Part model, mm, in its own coordinate system. A direction names the side the tool comes from. Coordinates: 2 decimals unless noted, no trailing zeros. Loops run counter-clockwise (first coordinate to the right, second up) from the corner with the lowest first, then second, coordinate; pieces in that order, holes last. Notation, with made-up numbers: M 12.25,76 L 52.25,76 A12 ccw 52.25,82 Z; hole C 51.5,57 d2. An arc over 180 degrees is marked long. Answer as a JSON object with one key per item and string values. Group by question number.
1. Drill centre lines: L1, parallel to Z at x = 0.25, y = 46.5; L2, parallel to X at y = 78.5, z = -4.5; L3, parallel to Y at x = -6, z = 2.5. Where is each one in solid material? Low to high.
2. Mould opens along X. For faces 1 (the face through (-6.083, 78.324, 6.633)), 2 (the face through (0, -1, 0)), 3 (the face through (2.465, 82.042, 4.35)) say: released by +X, released by -X, zero draft, split by the parting line, or undercut.
3. Drop flat-ended pins along their axis: pin 1 Ø10 at (y, z) = (54, -4) entering from +X; pin 2 Ø3 at (y, z) = (34, -3) entering from +X; pin 3 Ø2 at (y, z) = (60.5, 3.5) entering from +X. Give the stop position or say it passes through.
4. Saw through at A-A on y = 20. Write the cut outline in (x, z).
5. 3-axis set-ups, long thin cutter, end or side, ignore diameter. For faces 4 (the face through (6, 73, -2)), 5 (the face through (-2.535, 82.042, 4.31)), 6 (the face through (2, 85, 5)): which of +Z, -Z, +X, -X, +Y, -Y reach the whole face in a straight line?
from build123d import *
from build123d.topology import SkipClean

# Parameters (mm, degrees)
CUT_EXTRUDE1_DEPTH = 6


# Read off the part's stored shape, not the designer's step: Move Face1
with BuildPart() as part:
    # Sketch1 → Revolve1 (revolve)
    with BuildSketch(Plane(origin=(0, 0, 0), x_dir=(0, 0, -1), z_dir=(1, 0, 0)), mode=Mode.PRIVATE) as revolve1_sk:
        with BuildLine():
            Line((0, 78.118365096), (-5, 79))
            Line((-5, 79), (-5, 85))
            Line((-5, 85), (-7.8, 85))
            ThreePointArc((-7.8, 85), (-8.648528137, 84.648528137), (-9, 83.8))
            Line((-9, 83.8), (-9, 73))
            Line((-9, 73), (-6, 73))
            Line((-6, 73), (-6, 1.2))
            Line((-6, 1.2), (-4.8, 0))
            Line((-4.8, 0), (0, 0))
            Line((0, 0), (0, 78.118365096))
        make_face()
    revolve(revolve1_sk.sketch.rotate(Axis((0, 0, 0), (0, 1, 0)), 180), axis=Axis((0, 0, 0), (0, 1, 0)))

    # Sketch2 → Cut-Extrude1 (cut)
    with BuildSketch(Plane(origin=(0, 85, 0), x_dir=(1, 0, 0), z_dir=(0, 1, 0))):
        Polygon((0, 5.773502692), (-5, 2.886751346), (-5, -2.886751346), (0, -5.773502692), (5, -2.886751346), (5, 2.886751346), align=None)
    extrude(amount=-CUT_EXTRUDE1_DEPTH, mode=Mode.SUBTRACT)

    # Move Face1 outline → Move Face1 (revolve)
    with SkipClean():  # the faces are left unmerged after this step: merging them gives an invalid solid
        with BuildSketch(Plane.XY):
            Polygon((0, -1), (4.8, -1), (6, 0.2), (6, 1.2), (4.8, 0), (0, 0), align=None)
        revolve(axis=Axis((0, 0, 0), (0, 1, 0)))
    add(part.part.scale(1), mode=Mode.REPLACE)  # the faces are merged on a copy


solid = part.part
Outcome:
{
 "1": {"L1": "z = -5.99 to 5.99", "L2": "x = -7.79 to 7.79", "L3": "y = 73 to 85"},
 "2": {"face 1": "split by the parting line", "face 2": "zero draft", "face 3": "undercut"},
 "3": {"pin 1": "stops at x = 6", "pin 2": "stops at x = 5.81", "pin 3": "stops at x = 5.45"},
 "4": {"outline": "C 0,0 d12"},
 "5": {"face 4": "-Y", "face 5": "+Y", "face 6": "+Z, -Z, +X, -X, +Y"}
}
